Check sheet for the modelled part. Datum: model origin and axes. Units: mm. A direction names the side the tool comes from. Round coordinates to 2 decimals unless told otherwise and drop trailing zeros. Order: outer loops, then holes, each group sorted by start corner. A loop starts at its lowest first (then second) coordinate and runs counter-clockwise, first axis right, second up.
from build123d import *

# Parameters (mm, degrees)
BOSS_EXTRUDE1_DEPTH   = 34.6075
CUT_EXTRUDE1_START    = -4.7625
CUT_EXTRUDE1_DEPTH    = 4.7625
CUT_EXTRUDE2_START    = 9.525
CUT_EXTRUDE2_DEPTH    = 4.7625
CUT_EXTRUDE3_START    = -4.7625
CUT_EXTRUDE3_DEPTH    = 40.64
BOSS_EXTRUDE3_START   = 34.6075
SKETCH7_W             = 9.525
SKETCH7_H             = 6.35
BOSS_EXTRUDE3_DEPTH   = 69.215
FILLET1_R             = 3.175
FILLET2_R             = 2.38125
FILLET3_R             = 2.38125
BOSS_EXTRUDE4_DEPTH   = 9.525
CUT_EXTRUDE4_DEPTH    = 42.40423997
FILLET4_R             = 3.175
FILLET5_R             = 9.525
F_4_CLEARANCE_HOLE1_D = 3.2639


with BuildPart() as part:
    # Sketch1 → Boss-Extrude1 (new, symmetric)
    with BuildSketch(Plane.XY):
        with BuildLine():
            Line((-4.7625, 0), (4.7625, 0))
            Line((4.7625, 0), (4.7625, -15.875))
            ThreePointArc((4.7625, -15.875), (0, -20.6375), (-4.7625, -15.875))
            Line((-4.7625, -15.875), (-4.7625, 0))
        make_face()
    extrude(amount=BOSS_EXTRUDE1_DEPTH, both=True)

    # Sketch2 → Cut-Extrude1 (cut)
    with BuildSketch(Plane.XY.offset(34.6075).offset(CUT_EXTRUDE1_START)):
        with BuildLine():
            Line((-4.7625, -15.875), (-4.7625, -6.35))
            Line((-4.7625, -6.35), (4.7625, -6.35))
            Line((4.7625, -6.35), (4.7625, -15.875))
            ThreePointArc((4.7625, -15.875), (0, -20.6375), (-4.7625, -15.875))
        make_face()
    extrude(amount=-CUT_EXTRUDE1_DEPTH, mode=Mode.SUBTRACT)

    # Sketch3 → Cut-Extrude2 (cut)
    with BuildSketch(Plane.XY.offset(-34.6075).offset(CUT_EXTRUDE2_START)):
        with BuildLine():
            Line((-4.7625, -15.875), (-4.7625, -6.35))
            Line((-4.7625, -6.35), (4.7625, -6.35))
            Line((4.7625, -6.35), (4.7625, -15.875))
            ThreePointArc((4.7625, -15.875), (0, -20.6375), (-4.7625, -15.875))
        make_face()
    extrude(amount=-CUT_EXTRUDE2_DEPTH, mode=Mode.SUBTRACT)

    # Sketch5 → Cut-Extrude3 (cut)
    with BuildSketch(Plane.XY.offset(25.0825).offset(CUT_EXTRUDE3_START)):
        with BuildLine():
            Line((4.7625, -15.875), (4.7625, 0))
            Line((4.7625, 0), (-4.7625, 0))
            Line((-4.7625, 0), (-4.7625, -15.875))
            ThreePointArc((-4.7625, -15.875), (0, -20.6375), (4.7625, -15.875))
        make_face()
    extrude(amount=-CUT_EXTRUDE3_DEPTH, mode=Mode.SUBTRACT)


with BuildPart() as cut_extrude3_piece_1:
    # of the separate pieces the step leaves, piece 1, a body of its own (cut_extrude3_pieces)
    add(part.part.solids().sort_by_distance((-4.7625, 0, 20.32))[0])



with BuildPart() as cut_extrude3_piece_2:
    # of the separate pieces the step leaves, piece 2, a body of its own (cut_extrude3_pieces)
    add(part.part.solids().sort_by_distance((-4.7625, -15.875, -34.6075))[0])


with BuildPart() as cut_extrude3_piece_1_1:
    add(cut_extrude3_piece_1.part)

    add(cut_extrude3_piece_2.part)  # Boss-Extrude3 merges Cut-Extrude3 piece 2
    # Sketch7 → Boss-Extrude3 (add)
    with BuildSketch(Plane.XY.offset(BOSS_EXTRUDE3_START)):
        with Locations((0, 3.175)):
            Rectangle(SKETCH7_W, SKETCH7_H)
    extrude(amount=-BOSS_EXTRUDE3_DEPTH)

    # Fillet1
    fillet1_edges = [cut_extrude3_piece_1_1.edges().sort_by_distance(p)[0] for p in [
        (0, 0, 20.32),
        (0, 0, -20.32),
    ]]
    fillet(fillet1_edges, radius=FILLET1_R)

    # Fillet2
    fillet2_edges = [cut_extrude3_piece_1_1.edges().sort_by_distance(p)[0] for p in [
        (0, -6.35, -25.0825),
        (0, -6.35, -29.845),
    ]]
    fillet(fillet2_edges, radius=FILLET2_R - 0.0001)  # a hair under: the kernel refuses the full size

    # Fillet3
    fillet3_edges = [cut_extrude3_piece_1_1.edges().sort_by_distance(p)[0] for p in [
        (0, -6.35, 29.845),
        (0, -6.35, 25.0825),
    ]]
    fillet(fillet3_edges, radius=FILLET3_R - 0.0001)  # a hair under: the kernel refuses the full size

    # Sketch8 → Boss-Extrude4 (add)
    with BuildSketch(Plane.ZY.offset(4.7625)):
        with BuildLine():
            Line((-14.549677831, 6.35), (14.549677831, 6.35))
            ThreePointArc((14.549677831, 6.35), (0, 15.875), (-14.549677831, 6.35))
        make_face()
    extrude(amount=-BOSS_EXTRUDE4_DEPTH)

    # Sketch9 → Cut-Extrude4 (cut, through all)
    with BuildSketch(Plane.ZY.offset(4.7625)):
        with BuildLine():
            Line((-7.9375, 0), (7.9375, 0))
            ThreePointArc((7.9375, 0), (0, 7.9375), (-7.9375, 0))
        make_face()
    extrude(amount=-CUT_EXTRUDE4_DEPTH, mode=Mode.SUBTRACT)

    # Fillet4
    fillet4_edges = [cut_extrude3_piece_1_1.edges().sort_by_distance(p)[0] for p in [
        (0, 6.35, -14.549677831),
        (0, 6.35, 14.549677831),
        (0, 0, -7.9375),
        (0, 0, 7.9375),
    ]]
    fillet(fillet4_edges, radius=FILLET4_R)

    # Fillet5
    fillet5_edges = [cut_extrude3_piece_1_1.edges().sort_by_distance(p)[0] for p in [
        (0, 6.35, 34.6075),
        (0, 6.35, -34.6075),
    ]]
    fillet(fillet5_edges, radius=FILLET5_R)

    # #4 Clearance Hole1 (through all)
    with Locations(Plane(origin=(0, 0, -34.6075), x_dir=(-1, 0, 0), z_dir=(0, 0, -1))):
        with Locations((0, -14.2875)):
            Hole(F_4_CLEARANCE_HOLE1_D / 2)


solid = cut_extrude3_piece_1_1.part
1) Draft check along X on faces 3 (the face through (0, 0, 14)), 4 (the face through (-0.35, -15.88, 22.73)), 5 (the face through (-0.35, -15.88, -32.19)), 6 (the face through (0.105, -20.636, -22.668)). Enter one of: pulls with the +X half, pulls with the -X half, needs draft (parallel to the pull), parting line crosses it, or undercut.
2) Sectioned sample at A-A on y = -11. Record the cut outline in (x, z) (1 decimal).
3) Sectioned sample at C-C on x = 0. Count the separate pieces of the cut face and the enclosed holes in it, and give its area (3 significant figures).
4) Sectioned sample at B-B on y = -5. Record the cut outline in (x, z), and give its area (3 significant figures).
5) Scan lines: line 1 (Z direction, x = 1.5, y = -10) (1 decimal); line 2 (Y direction, x = 0, z = 23.7); line 3 (Y direction, x = 0, z = 33.2). Record each from-to range of solid material in increasing order.
6) Gauge pin test, flat ends, axial feed: pin 1 (1.9 mm diameter, centred on x = -2.5, z = -13, fed in from -Y); pin 2 (12 mm diameter, centred on y = -2.5, z = 2.5, fed in from +X); pin 3 (2.5 mm diameter, centred on x = -2, z = 21.5, fed in from +Y). Record the tip position at first contact, or that the pin passes through.
7) Set-up check for faces 1 (the face through (0.105, -20.636, 22.735)), 2 (the face through (0.067, 0.612, -8.775)): record each of +Z, -Z, +X, -X, +Y, -Y from which the full face is reachable in a straight line by a thin tool's end or side.
Values found:
1. face 3: needs draft
1. face 4: undercut
1. face 5: undercut
1. face 6: parting line crosses it
2. outline: (-4.8, -34.6) - (4.8, -34.6) - (4.8, -29.8) - (-4.8, -29.8) - close; (-4.8, -25.1) - (4.8, -25.1) - (4.8, -20.3) - (-4.8, -20.3) - close; (-4.8, 20.3) - (4.8, 20.3) - (4.8, 25.1) - (-4.8, 25.1) - close; (-4.8, 29.8) - (4.8, 29.8) - (4.8, 34.6) - (-4.8, 34.6) - close
3. separate pieces: 5
3. enclosed holes: 0
3. area: 901 mm2
4. outline: (-4.76, -34.61) - (4.76, -34.61) - (4.76, -20.32) - (-4.76, -20.32) - close; (-4.76, 20.32) - (4.76, 20.32) - (4.76, 34.61) - (-4.76, 34.61) - close
4. area: 272 mm2
5. line 1: z = -34.6 to -29.8, -25.1 to -20.3, 20.3 to 25.1, 29.8 to 34.6
5. line 2: y = -20.64 to -15.92, -12.66 to 6.35
5. line 3: y = -20.64 to -15.92, -12.66 to 1.81
6. pin 1: stops at y = 0
6. pin 2: passes through
6. pin 3: stops at y = 6.35
7. face 1: +Z, -Z, -Y
7. face 2: +X, -X, -Y
